from build123d import *

# Parameters (mm, degrees)
SKETCH_1_R          = 3.5
EXTRUDE_1_DEPTH     = 25
SKETCH_2_R          = 1.5
EXTRUDE_2_DEPTH     = 10
SKETCH_3_W          = 2
SKETCH_3_H          = 2
EXTRUDE_3_DEPTH     = 3.5
SKETCH_4_OUTSIDE_W  = 16.95
SKETCH_4_OUTSIDE_H  = 16.95
SKETCH_4_OUTSIDE_R  = 2.5
CUT_EXTRUDE_1_DEPTH = 20
SKETCH_5_W          = 1.5
SKETCH_5_H          = 0.547111854
CUT_EXTRUDE_2_DEPTH = 11.820119966


with BuildPart() as part:
    # 草图1 → 拉伸1 (new body)
    with BuildSketch(Plane.XY):
        Circle(SKETCH_1_R)
    extrude(amount=EXTRUDE_1_DEPTH)

    # 草图2 → 拉伸2 (add)
    with BuildSketch(Plane(origin=(0, 0, 0), x_dir=(-1, 0, 0), z_dir=(0, 0, -1))):
        with Locations(Location((0, 0, 0), (0, 0, 180))):
            Circle(SKETCH_2_R)
    extrude(amount=EXTRUDE_2_DEPTH)

    # 草图3 → 拉伸3 (add)
    with BuildSketch(Plane(origin=(0, 0, -10), x_dir=(-1, 0, 0), z_dir=(0, 0, -1))):
        Rectangle(SKETCH_3_W, SKETCH_3_H)
    extrude(amount=EXTRUDE_3_DEPTH)

    # 草图4 outside → 切除-拉伸1 (cut)
    with BuildSketch(Plane.XY.offset(25)):
        Rectangle(SKETCH_4_OUTSIDE_W, SKETCH_4_OUTSIDE_H)
        Circle(SKETCH_4_OUTSIDE_R, mode=Mode.SUBTRACT)
    extrude(amount=-CUT_EXTRUDE_1_DEPTH, mode=Mode.SUBTRACT)

    # 草图5 → 切除-拉伸2 (cut)
    with BuildSketch(Plane.XY.offset(25)):
        with Locations((0, 2.491129658)):
            Rectangle(SKETCH_5_W, SKETCH_5_H)
    extrude(amount=-CUT_EXTRUDE_2_DEPTH, mode=Mode.SUBTRACT)


solid = part.part
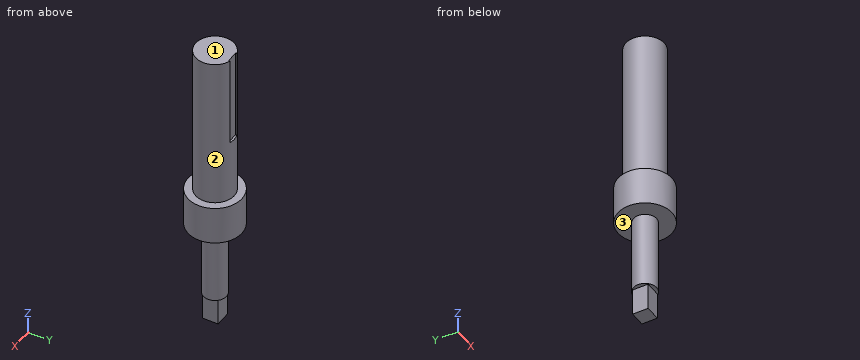
Here's how the part is built. I have some questions about the finished solid (model axes, mm). Face numbers are marked on the shaded views. A direction names the side the tool comes from. Round coordinates to 2 decimals unless told otherwise and drop trailing zeros. Write each loop counter-clockwise with the first axis right and the second up, starting at its lowest first coordinate (ties: lowest second). Pieces come first, ordered by that corner, then holes. Notation, with made-up numbers: (84.25, -14.75) -> (89.25, -14.75) arc R16 cw to (89.25, 11.25) -> close; hole circle Ø6 at (18.25, 29.25). An arc over 180 degrees is marked (long way). One line per item, written item: value.
1) I'm going to push flat-ended pins straight in: pin 1 Ø1.2 at (x, z) = (0, 21) entering from +Y; pin 2 Ø1 at (y, z) = (0, -11) entering from +X; pin 3 Ø3 at (y, z) = (-2, 20.5) entering from +X. Where does each tip first touch, or does it pass through?
Filled sheet:
pin 1: stops at y = 2.22
pin 2: stops at x = 1
pin 3: stops at x = 2.45
2) For the marked faces 1, 2 and 3, which set-ups out of +Z, -Z, +X, -X, +Y, -Y let a thin tool reach every point of the face, with its end or its side?
Filled sheet:
face 1: +Z, +X, -X, +Y, -Y
face 2: +Z
face 3: -Z
3) Suppose I cut it at B-B on x = 0. List the corners of the cut face in (y, z) for me.
Filled sheet:
outline: (-3.5, 0) -> (-1.5, 0) -> (-1.5, -10) -> (-1, -10) -> (-1, -13.5) -> (1, -13.5) -> (1, -10) -> (1.5, -10) -> (1.5, 0) -> (3.5, 0) -> (3.5, 5) -> (2.5, 5) -> (2.5, 13.18) -> (2.22, 13.18) -> (2.22, 25) -> (-2.5, 25) -> (-2.5, 5) -> (-3.5, 5) -> close
4) If I drill on line 1 (Z direction, x = 0.5, y = -1.5); line 2 (Z direction, x = 2.5, y = -0.5); line 3 (Y direction, x = 0, z = -8), over which ranges is the centre line in solid material (lowest first)? Write a range as [from, to].
Filled sheet:
line 1: z = [0, 25]
line 2: z = [0, 5]
line 3: y = [-1.5, 1.5]
5) Suppose I cut it at A-A on y = 0. List the corners of the cut face in (x, z) for me, plus the area to 3 significant figures.
Filled sheet:
outline: (-3.5, 0) -> (-1.5, 0) -> (-1.5, -10) -> (-1, -10) -> (-1, -13.5) -> (1, -13.5) -> (1, -10) -> (1.5, -10) -> (1.5, 0) -> (3.5, 0) -> (3.5, 5) -> (2.5, 5) -> (2.5, 25) -> (-2.5, 25) -> (-2.5, 5) -> (-3.5, 5) -> close
area: 172 mm2
6) Suppose I cut it at C-C on z = 23. List the corners of the cut face in (x, y) for me, plus the area to 3 significant figures.
Filled sheet:
outline: (-0.75, 2.22) -> (-0.75, 2.38) arc R2.5 ccw (long way) to (0.75, 2.38) -> (0.75, 2.22) -> close
area: 19.3 mm2
